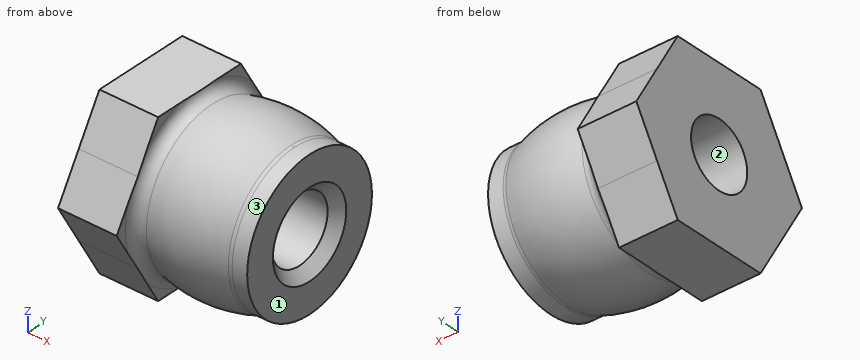
```python
from build123d import *

# Parameters (mm, degrees)
BOSS_EXTRUDE1_START = -2.2225
SKETCH2_R           = 3.175
SKETCH2_R_2         = 1.2446
BOSS_EXTRUDE1_DEPTH = 2.2225
SKETCH3_R           = 2.76225
SKETCH3_R_2         = 1.2446
BOSS_EXTRUDE2_DEPTH = 0.635
FILLET1_R           = 0.381
FILLET2_R           = 0.381
CHAMFER1_SIZE       = 0.381


with BuildPart() as part:
    # Sketch1 → Revolve1 (revolve)
    with BuildSketch(Plane.XY, mode=Mode.PRIVATE) as revolve1_sk:
        with BuildLine():
            Line((0, 1.2446), (-5.7531, 1.2446))
            Line((-5.7531, 1.2446), (-5.7531, 3.175))
            Line((-5.7531, 3.175), (-3.5306, 3.175))
            Line((-3.5306, 3.175), (-3.5306, 2.76225))
            ThreePointArc((-3.5306, 2.76225), (-1.7653, 3.078835688), (0, 2.76225))
            Line((0, 2.76225), (0, 1.2446))
        make_face()
    revolve(revolve1_sk.sketch.rotate(Axis((-60.338913039, 0, 0), (1, 0, 0)), 90), axis=Axis((-60.338913039, 0, 0), (1, 0, 0)))

    # Sketch2 → Boss-Extrude1 (add)
    # profile 1 of 7: a face of its own
    with BuildSketch(Plane.ZY.offset(5.7531).offset(BOSS_EXTRUDE1_START)):
        with BuildLine():
            ThreePointArc((-1.587499996, 2.749630659), (1.5e-08, 3.175), (1.587500022, 2.749630644))
            Line((1.587500022, 2.749630644), (0, 3.666174209))
            Line((0, 3.666174209), (-1.587499996, 2.749630659))
        make_face()
    # profile 2 of 7: a face of its own
    with BuildSketch(Plane.ZY.offset(5.7531).offset(BOSS_EXTRUDE1_START)):
        with BuildLine():
            ThreePointArc((1.587500022, 2.749630644), (2.749630663, 1.587499989), (3.175, 0))
            Line((3.175, 0), (3.175, 1.833087105))
            Line((3.175, 1.833087105), (1.587500022, 2.749630644))
        make_face()
    # profile 3 of 7: a face of its own
    with BuildSketch(Plane.ZY.offset(5.7531).offset(BOSS_EXTRUDE1_START)):
        with BuildLine():
            Line((1.587500022, -2.749630644), (3.175, -1.833087105))
            Line((3.175, -1.833087105), (3.175, 0))
            ThreePointArc((3.175, 0), (2.749630663, -1.587499989), (1.587500022, -2.749630644))
        make_face()
    # profile 4 of 7: a face of its own
    with BuildSketch(Plane.ZY.offset(5.7531).offset(BOSS_EXTRUDE1_START)):
        with BuildLine():
            Line((0, -3.666174209), (1.587500022, -2.749630644))
            ThreePointArc((1.587500022, -2.749630644), (3.9e-08, -3.175), (-1.587499954, -2.749630684))
            Line((-1.587499954, -2.749630684), (0, -3.666174209))
        make_face()
    # profile 5 of 7: a face of its own
    with BuildSketch(Plane.ZY.offset(5.7531).offset(BOSS_EXTRUDE1_START)):
        with BuildLine():
            Line((-3.175, -1.833087105), (-1.587499954, -2.749630684))
            ThreePointArc((-1.587499954, -2.749630684), (-2.749630644, -1.587500023), (-3.175, 0))
            Line((-3.175, 0), (-3.175, -1.833087105))
        make_face()
    # profile 6 of 7: a face of its own
    with BuildSketch(Plane.ZY.offset(5.7531).offset(BOSS_EXTRUDE1_START)):
        with BuildLine():
            ThreePointArc((-3.175, 0), (-2.749630656, 1.587500002), (-1.587499996, 2.749630659))
            Line((-1.587499996, 2.749630659), (-3.175, 1.833087105))
            Line((-3.175, 1.833087105), (-3.175, 0))
        make_face()
    # profile 7 of 7: a face of its own
    with BuildSketch(Plane.ZY.offset(5.7531).offset(BOSS_EXTRUDE1_START)):
        Circle(SKETCH2_R)
        Circle(SKETCH2_R_2, mode=Mode.SUBTRACT)
    extrude(amount=BOSS_EXTRUDE1_DEPTH)

    # Sketch3 → Boss-Extrude2 (add)
    with BuildSketch(Plane(origin=(0, 0, 0), x_dir=(0, 0, -1), z_dir=(1, 0, 0))):
        Circle(SKETCH3_R)
        with Locations(Location((0, 0, 0), (0, 0, 180))):
            Circle(SKETCH3_R_2, mode=Mode.SUBTRACT)
    extrude(amount=BOSS_EXTRUDE2_DEPTH)

    # Fillet1
    # the kernel refuses this fillet: 0.381 mm, written as the material it adds along each edge
    with BuildSketch(Plane(origin=(-3.5306, 0, 0), x_dir=(0, 0, 1), z_dir=(0, 1, 0))) as fillet1_piece_1_section:
        with BuildLine():
            CenterArc((3.281470874, 0.381), FILLET1_R, 165.315967452, 104.684032548)
            Line((3.281470874, 0), (2.76225, 0))
            ThreePointArc((2.76225, 0), (2.84347095, 0.236931857), (2.912914931, 0.47757907))
        make_face()
    fillet1_piece_1 = revolve(axis=Axis((-3.5306, 0, 0), (1, 0, 0)), mode=Mode.PRIVATE)
    fillet1_piece_1 = split(fillet1_piece_1, bisect_by=Plane(origin=(-3.388915245, -4.036268752, -0.641022551), z_dir=(0, 0.8660254037844388, -0.49999999999999983)), keep=Keep.TOP, mode=Mode.PRIVATE)
    fillet1_piece_1 = split(fillet1_piece_1, bisect_by=Plane(origin=(-3.388915245, -1.462992562, -3.816022551), z_dir=(0, 0.8660254037844387, 0.5)), keep=Keep.TOP, mode=Mode.PRIVATE)
    fillet1_piece_1 = split(fillet1_piece_1, bisect_by=Plane(origin=(-3.388915245, 0, -3.175), z_dir=(0, 0, 1)), keep=Keep.TOP, mode=Mode.PRIVATE)
    fillet1_piece_1 = split(fillet1_piece_1, bisect_by=Plane(origin=(-3.388915245, 1.462992562, -3.816022551), z_dir=(0, -0.8660254037844387, 0.49999999999999994)), keep=Keep.TOP, mode=Mode.PRIVATE)
    fillet1_piece_1 = split(fillet1_piece_1, bisect_by=Plane(origin=(-3.388915245, 4.036268752, -0.641022551), z_dir=(0, -0.8660254037844387, -0.49999999999999983)), keep=Keep.TOP, mode=Mode.PRIVATE)
    fillet1_piece_1 = split(fillet1_piece_1, bisect_by=Plane(origin=(-3.388915245, 0, 3.175), z_dir=(0, 0, -1)), keep=Keep.TOP, mode=Mode.PRIVATE)
    add(fillet1_piece_1)

    # Fillet2
    fillet2_edges = [part.edges().sort_by_distance(p)[0] for p in [
        (0, -2.76225, 0),
    ]]
    fillet(fillet2_edges, radius=FILLET2_R)

    # Chamfer1
    chamfer1_edges = [part.edges().sort_by_distance(p)[0] for p in [
        (0.635, 0, -1.2446),
    ]]
    chamfer(chamfer1_edges, length=CHAMFER1_SIZE)


solid = part.part
```
Read the model definition and answer for the solid it produces. Units are mm, in the model's axes. Face numbers are marked on the shaded views. Give positions to 0.01 mm unless a question says otherwise; leave off trailing zeros. Write each loop counter-clockwise with the first axis right and the second up, starting at its lowest first coordinate (ties: lowest second). Pieces come first, ordered by that corner, then holes. Notation, with made-up numbers: (20.25, -7) -> (64.25, -7) arc R22 cw to (64.25, 9) -> close; hole circle Ø11 at (81.25, 3.5). An arc over 180 degrees is marked (long way). Answer as a JSON object with one key per item and string values.
1) For a pull along Y with two mould halves and no side action, classify the marked faces 1, 2 and 3 as pulls with the +Y half, pulls with the -Y half, needs draft (parallel to the pull), parting line crosses it, or undercut.
Findings below:
{"face 1": "needs draft", "face 2": "undercut", "face 3": "parting line crosses it"}
2) Section A-A on x = -3.25 is taken. Write down the section's boundary in (y, z).
Findings below:
{"outline": "circle Ø5.83 at (0, 0); hole circle Ø2.49 at (0, 0)"}
3) Straight lines are drawn through the part: probe 1 along X at (y, z) = (-2, 2.75); probe 2 along Y at (x, z) = (-4.5, 1); probe 3 along Y at (x, z) = (-2.25, 0). For each, find the intervals that lie inside material, in ascending order. Write a range as from..to.
Findings below:
{"probe 1": "x = -5.75..-3.53", "probe 2": "y = -3.09..-0.74, 0.74..3.09", "probe 3": "y = -3.06..-1.24, 1.24..3.06"}
4) Flat-ended cylindrical pins translate along their axes: pin 1 Ø3 at (x, z) = (-1, 2.5) entering from -Y; pin 2 Ø2 at (x, z) = (-3, -2) entering from +Y; pin 3 Ø0.6 at (y, z) = (-3.5, 0.5) entering from +X. Find the tip coordinate at first contact, or state that the pin passes through.
Findings below:
{"pin 1": "stops at y = -2.88", "pin 2": "stops at y = 3", "pin 3": "stops at x = -3.53"}
